```python
from build123d import *

# Parameters (mm, degrees)
EXTRUDE_1_DEPTH      = 50
SKETCH_2_W           = 50
SKETCH_2_H           = 10
EXTRUDE_2_DEPTH      = 10
SKETCH_3_W           = 10
SKETCH_3_H           = 20
EXTRUDE_3_DEPTH      = 20
SKETCH_4_W           = 20
SKETCH_4_H           = 10
EXTRUDE_4_DEPTH      = 30
CUT_EXTRUDE_1_DEPTH  = 50
CHAMFER_1_SIZE       = 2
SKETCH_9_R           = 1.5
CUT_EXTRUDE_2_DEPTH  = 66.493778942
CUT_EXTRUDE_4_DEPTH  = 6
SKETCH_13_W          = 4
SKETCH_13_H          = 6
EXTRUDE_12_DEPTH     = 18
SKETCH_14_W          = 20
SKETCH_14_H          = 20
EXTRUDE_13_DEPTH     = 6
CUT_EXTRUDE_START    = -20
SKETCH_15_W          = 50
SKETCH_15_H          = 6
CUT_EXTRUDE_5_DEPTH  = 20
SKETCH_16_W          = 4
SKETCH_16_H          = 4
CUT_EXTRUDE_7_DEPTH  = 18
EXTRUDE_14_REACH     = 68.163
SKETCH_17_W          = 5
SKETCH_17_H          = 30
SKETCH_18_W          = 50
SKETCH_18_H          = 4
EXTRUDE_15_DEPTH     = 18
CUT_EXTRUDE_8_REACH  = 67.494
SKETCH_19_W          = 60
SKETCH_19_H          = 10
SKETCH_20_R          = 1.5
CUT_EXTRUDE_9_DEPTH  = 4
CHAMFER_2_SIZE       = 2
SKETCH_21_W          = 15
SKETCH_21_H          = 50
CUT_EXTRUDE_10_DEPTH = 10
SKETCH_22_W          = 5
SKETCH_22_H          = 50
EXTRUDE_16_DEPTH     = 19
SKETCH_23_W          = 7
SKETCH_23_H          = 50
CUT_EXTRUDE_11_DEPTH = 4.2
EXTRUDE_17_DEPTH     = 3
SKETCH_25_R          = 1.5
CUT_EXTRUDE_12_DEPTH = 8
SKETCH_26_R          = 2.9
CUT_EXTRUDE_13_DEPTH = 6
CUT_EXTRUDE_14_REACH = 67.988
SKETCH_27_W          = 4
SKETCH_27_H          = 10
SKETCH_29_W          = 8
SKETCH_29_H          = 10
EXTRUDE_18_DEPTH     = 6
SKETCH_30_W          = 50
SKETCH_30_H          = 5
CUT_EXTRUDE_15_DEPTH = 4
EXTRUDE_19_REACH     = 75.219
SKETCH_31_W          = 9.8
SKETCH_31_H          = 10


with BuildPart() as part:
    # 草图1 → 凸台-拉伸1 (new body)
    with BuildSketch(Plane(origin=(0, 0, 0), x_dir=(0, 0, -1), z_dir=(1, 0, 0))):
        Polygon((0, 0), (-10, 0), (-17.716362436, 40), (-12, 41.102738109), (-6, 10), (0, 10), align=None)
    extrude(amount=EXTRUDE_1_DEPTH)

    # 草图2 → 凸台-拉伸2 (add)
    with BuildSketch(Plane.XZ):
        with Locations((25, 5)):
            Rectangle(SKETCH_2_W, SKETCH_2_H)
    extrude(amount=EXTRUDE_2_DEPTH)

    # 草图3 → 凸台-拉伸3 (add)
    with BuildSketch(Plane.ZY):
        with Locations((5, 0)):
            Rectangle(SKETCH_3_W, SKETCH_3_H)
    extrude(amount=EXTRUDE_3_DEPTH)

    # 草图4 → 凸台-拉伸4 (add)
    with BuildSketch(Plane(origin=(0, 10, 0), x_dir=(1, 0, 0), z_dir=(0, 1, 0))):
        with Locations((-10, -5)):
            Rectangle(SKETCH_4_W, SKETCH_4_H)
    extrude(amount=EXTRUDE_4_DEPTH)

    # 草图5 → 切除-拉伸1 (cut)
    with BuildSketch(Plane(origin=(50, 0, 0), x_dir=(0, 0, -1), z_dir=(1, 0, 0))):
        Polygon((-10, 10), (-11.929090609, 10), (-10, 0), align=None)
    extrude(amount=-CUT_EXTRUDE_1_DEPTH, mode=Mode.SUBTRACT)

    # 倒角1
    # the kernel refuses this chamfer: 2 mm, written as the material it adds along each edge
    with BuildSketch(Plane(origin=(50, 10, 10), x_dir=(0, 0.027495876610586487, 0.9996219169112968), z_dir=(-1, 0, 0))) as chamfer_1_piece_1_section:
        Polygon((CHAMFER_1_SIZE * 0.999621916911, -CHAMFER_1_SIZE * 0.0274958766106), (-CHAMFER_1_SIZE * 0.0274958766106, -CHAMFER_1_SIZE * 0.999621916911), (0, 0), align=None)
    chamfer_1_piece_1 = extrude(amount=50, mode=Mode.PRIVATE)
    chamfer_1_piece_1 = split(chamfer_1_piece_1, bisect_by=Plane(origin=(25, 9.122791872, 11.759869213), z_dir=(0, 0.18941678522713282, -0.9818967774029093)), keep=Keep.TOP, mode=Mode.PRIVATE)
    add(chamfer_1_piece_1)

    # 草图9 → 切除-拉伸2 (cut, through all)
    with BuildSketch(Plane.XY.offset(10)):
        with Locations((-10, 30)):
            Circle(SKETCH_9_R)
        with Locations((30, 0)):
            Circle(SKETCH_9_R)
    extrude(amount=-CUT_EXTRUDE_2_DEPTH, mode=Mode.SUBTRACT)

    # 草图12 → 切除-拉伸4 (cut)
    with BuildSketch(Plane.XY.offset(10)):
        Polygon((0, 30.73515874), (0, 40), (-20, 40), (-20, -10), (50, -10), (50, 8), (0, 8), align=None)
    extrude(amount=-CUT_EXTRUDE_4_DEPTH, mode=Mode.SUBTRACT)

    # 草图13 → 凸台-拉伸12 (add)
    with BuildSketch(Plane.XZ.offset(-8)):
        with Locations((2, 7)):
            Rectangle(SKETCH_13_W, SKETCH_13_H)
        with Locations((48, 7)):
            Rectangle(SKETCH_13_W, SKETCH_13_H)
    extrude(amount=EXTRUDE_12_DEPTH)

    # 草图14 → 凸台-拉伸13 (add)
    with BuildSketch(Plane.XY.offset(4)):
        with Locations((-10, 0)):
            Rectangle(SKETCH_14_W, SKETCH_14_H)
    extrude(amount=EXTRUDE_13_DEPTH)

    # 草图15 → 切除-拉伸5 (cut)
    with BuildSketch(Plane(origin=(0, 10, 0), x_dir=(1, 0, 0), z_dir=(0, 1, 0)).offset(CUT_EXTRUDE_START)):
        with Locations((25, -3)):
            Rectangle(SKETCH_15_W, SKETCH_15_H)
    extrude(amount=CUT_EXTRUDE_5_DEPTH, mode=Mode.SUBTRACT)

    # 草图16 → 切除-拉伸7 (cut)
    with BuildSketch(Plane.XZ.offset(10)):
        with Locations((2, 8)):
            Rectangle(SKETCH_16_W, SKETCH_16_H)
        with Locations((48, 8)):
            Rectangle(SKETCH_16_W, SKETCH_16_H)
    extrude(amount=-CUT_EXTRUDE_7_DEPTH, mode=Mode.SUBTRACT)

    # 凸台-拉伸14: up to this plane
    extrude_14_end = Plane(origin=(50, 0, 10), z_dir=(0, 0.1894167852271328, -0.9818967774029093))
    # 草图17 → 凸台-拉伸14 (add, up to the surface)
    with BuildSketch(Plane.XY.offset(4), mode=Mode.PRIVATE) as extrude_14_sk1:
        with Locations((-2.5, 25)):
            Rectangle(SKETCH_17_W, SKETCH_17_H)
    extrude_14_tool1 = split(extrude(extrude_14_sk1.sketch, amount=EXTRUDE_14_REACH, mode=Mode.PRIVATE), bisect_by=extrude_14_end, keep=Keep.BOTH, mode=Mode.PRIVATE)
    add(extrude_14_tool1.solids().sort_by_distance((-2.5, 25, 4))[0])

    # 草图18 → 凸台-拉伸15 (add)
    with BuildSketch(Plane.XZ.offset(-8)):
        with Locations((25, 8)):
            Rectangle(SKETCH_18_W, SKETCH_18_H)
    extrude(amount=EXTRUDE_15_DEPTH)

    # 切除-拉伸8: up to this face of the body (flat: up to its plane)
    cut_extrude_8_end = Plane(part.part.faces().sort_by_distance((-12.539896603, 24.920206795, 4))[0])
    # 草图19 → 切除-拉伸8 (cut, up to the picked face)
    with BuildSketch(Plane.XY.offset(10), mode=Mode.PRIVATE) as cut_extrude_8_sk1:
        with Locations((10, 0)):
            Rectangle(SKETCH_19_W, SKETCH_19_H)
    cut_extrude_8_tool1 = split(extrude(cut_extrude_8_sk1.sketch, amount=-CUT_EXTRUDE_8_REACH, mode=Mode.PRIVATE), bisect_by=cut_extrude_8_end, keep=Keep.BOTH, mode=Mode.PRIVATE)
    add(cut_extrude_8_tool1.solids().sort_by(Axis((10, 0, 10), (0, 0, -1)))[0], mode=Mode.SUBTRACT)

    # 草图20 → 切除-拉伸9 (cut)
    with BuildSketch(Plane.XY.offset(4)):
        with Locations((-10, 0)):
            Circle(SKETCH_20_R)
    extrude(amount=-CUT_EXTRUDE_9_DEPTH, mode=Mode.SUBTRACT)

    # 倒角2
    # the kernel refuses this chamfer: 2 mm, written as the material it adds along each edge
    with BuildSketch(Plane(origin=(5.143365976, 10, 10), x_dir=(0, -0.9996219169112968, -0.027495876610586487), z_dir=(-1, 0, 0))) as chamfer_2_piece_1_section:
        Polygon((CHAMFER_2_SIZE * 0.999621916911, CHAMFER_2_SIZE * 0.0274958766106), (-CHAMFER_2_SIZE * 0.0274958766106, CHAMFER_2_SIZE * 0.999621916911), (0, 0), align=None)
    chamfer_2_piece_1 = extrude(amount=10.143365976, mode=Mode.PRIVATE)
    chamfer_2_piece_1 = split(chamfer_2_piece_1, bisect_by=Plane(origin=(-2.5, 9.121127045, 11.759548053), z_dir=(0, 0.18941678522698793, -0.9818967774029372)), keep=Keep.TOP, mode=Mode.PRIVATE)
    add(chamfer_2_piece_1)

    # 草图21 → 切除-拉伸10 (cut)
    with BuildSketch(Plane.XY.offset(10)):
        with Locations((-12.5, 15)):
            Rectangle(SKETCH_21_W, SKETCH_21_H)
    extrude(amount=-CUT_EXTRUDE_10_DEPTH, mode=Mode.SUBTRACT)

    # 草图22 → 凸台-拉伸16 (add)
    with BuildSketch(Plane(origin=(0, 0, 0), x_dir=(-1, 0, 0), z_dir=(0, 0, -1))):
        with Locations((2.5, 15)):
            Rectangle(SKETCH_22_W, SKETCH_22_H)
    extrude(amount=EXTRUDE_16_DEPTH)

    # 草图23 → 切除-拉伸11 (cut)
    with BuildSketch(Plane(origin=(0, 0, 0), x_dir=(0, 0, -1), z_dir=(1, 0, 0))):
        with Locations((15.5, 15)):
            Rectangle(SKETCH_23_W, SKETCH_23_H)
    extrude(amount=-CUT_EXTRUDE_11_DEPTH, mode=Mode.SUBTRACT)

    # 草图24 → 凸台-拉伸17 (add)
    with BuildSketch(Plane.ZY.offset(5)):
        Polygon((17.716362436, 40), (-19, 40), (-19, -10), (10, -10), (10, -5), (4, -5), (4, 5), (10, 5), (10, 8), (11.912142006, 9.912142006), align=None)
    extrude(amount=EXTRUDE_17_DEPTH)

    # 草图25 → 切除-拉伸12 (cut)
    with BuildSketch(Plane.ZY.offset(8)):
        with Locations(Location((-9, 30, 0), (0, 0, 270))):
            Circle(SKETCH_25_R)
        with Locations(Location((-9, 0, 0), (0, 0, 270))):
            Circle(SKETCH_25_R)
    extrude(amount=-CUT_EXTRUDE_12_DEPTH, mode=Mode.SUBTRACT)

    # 草图26 → 切除-拉伸13 (cut)
    with BuildSketch(Plane.ZY.offset(8)):
        with Locations(Location((-9, 30, 0), (0, 0, 270))):
            Circle(SKETCH_26_R)
        with Locations(Location((-9, 0, 0), (0, 0, 270))):
            Circle(SKETCH_26_R)
    extrude(amount=-CUT_EXTRUDE_13_DEPTH, mode=Mode.SUBTRACT)

    # 草图27 → 切除-拉伸14 (cut, up to next)
    with BuildSketch(Plane.ZY.offset(-40), mode=Mode.PRIVATE) as cut_extrude_14_sk1:
        with Locations((8, 0)):
            Rectangle(SKETCH_27_W, SKETCH_27_H)
    cut_extrude_14_tool1 = extrude(cut_extrude_14_sk1.sketch, amount=-CUT_EXTRUDE_14_REACH, mode=Mode.PRIVATE) & part.part
    add(cut_extrude_14_tool1.solids().sort_by_distance((40, 0, 8))[0], mode=Mode.SUBTRACT)

    # 草图29 → 凸台-拉伸18 (add)
    with BuildSketch(Plane.XY.offset(4)):
        with Locations((-4, 0)):
            Rectangle(SKETCH_29_W, SKETCH_29_H)
    extrude(amount=EXTRUDE_18_DEPTH)

    # 草图30 → 切除-拉伸15 (cut)
    with BuildSketch(Plane.XY.offset(10)):
        with Locations((25, -7.5)):
            Rectangle(SKETCH_30_W, SKETCH_30_H)
    extrude(amount=-CUT_EXTRUDE_15_DEPTH, mode=Mode.SUBTRACT)

    # 凸台-拉伸19: up to this face of the body (flat: up to its plane)
    extrude_19_end = Plane(part.part.faces().sort_by_distance((25, 5, 8))[0])
    # 草图31 → 凸台-拉伸19 (add, up to the picked face)
    with BuildSketch(Plane(origin=(0, 40, 0), x_dir=(1, 0, 0), z_dir=(0, 1, 0)), mode=Mode.PRIVATE) as extrude_19_sk1:
        with Locations((4.9, -7)):
            Rectangle(SKETCH_31_W, SKETCH_31_H)
    extrude_19_tool1 = split(extrude(extrude_19_sk1.sketch, amount=-EXTRUDE_19_REACH, mode=Mode.PRIVATE), bisect_by=extrude_19_end, keep=Keep.BOTH, mode=Mode.PRIVATE)
    add(extrude_19_tool1.solids().sort_by(Axis((4.9, 40, 7), (0, -1, 0)))[0])


solid = part.part
```
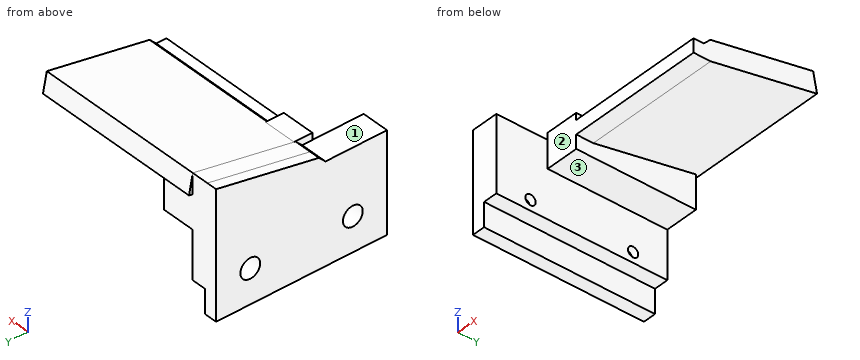
Verification items for the finished model (mm, model axes). Face numbers are marked on the shaded views. A direction names the side the tool comes from. Give positions to 0.01 mm unless a question says otherwise; leave off trailing zeros. Order: outer loops, then holes, each group sorted by start corner. A loop starts at its lowest first (then second) coordinate and runs counter-clockwise, first axis right, second up. Notation, with made-up numbers: (14, 51) -> (62, 51) arc R23 cw to (62, 72) -> close; hole circle Ø8 at (72.5, 56.25). An arc over 180 degrees is marked (long way). Use a Markdown table: item, result.
1) Depth check by flat-ended pin: pin 1 Ø4 at (y, z) = (-3, 13.5) entering from -X; pin 2 Ø11 at (x, z) = (19, 5) entering from -Y; pin 3 Ø6 at (x, y) = (6, 8) entering from +Z; pin 4 Ø0.9 at (y, z) = (40.5, 16) entering from -X. Enter the tip coordinate at first touch or a pass-through.
Results:
| item | result |
|---|---|
| pin 1 | through |
| pin 2 | y = 5 |
| pin 3 | z = 12.12 |
| pin 4 | x = 0 |
2) Section check B-B, the plane z = -9. Record the boundary of the cut face in (x, y), then the cut area to 3 significant figures.
Results:
| item | result |
|---|---|
| outline | (-8, -10) -> (0, -10) -> (0, -1.5) -> (-2, -1.5) -> (-2, -2.9) -> (-8, -2.9) -> close; (-8, 2.9) -> (-2, 2.9) -> (-2, 1.5) -> (0, 1.5) -> (0, 28.5) -> (-2, 28.5) -> (-2, 27.1) -> (-8, 27.1) -> close; (-8, 32.9) -> (-2, 32.9) -> (-2, 31.5) -> (0, 31.5) -> (0, 40) -> (-8, 40) -> close |
| area | 318 mm² |
3) Section check D-D, the plane z = 3.5. Record the boundary of the cut face in (x, y).
Results:
| item | result |
|---|---|
| outline | (-8, -10) -> (0, -10) -> (0, 5) -> (9.8, 5) -> (9.8, 40) -> (-8, 40) -> close |
4) Section check A-A, the plane y = 0. Record the boundary of the cut face in (x, z), then the cut area to 3 significant figures.
Results:
| item | result |
|---|---|
| outline | (-8, -19) -> (-4.2, -19) -> (-4.2, -12) -> (0, -12) -> (0, -10.5) -> (-2, -10.5) -> (-2, -11.9) -> (-8, -11.9) -> close; (-8, -6.1) -> (-2, -6.1) -> (-2, -7.5) -> (0, -7.5) -> (0, 10) -> (-8, 10) -> close |
| area | 162 mm² |
5) Section check C-C, the plane x = 36. Record the boundary of the cut face in (y, z).
Results:
| item | result |
|---|---|
| outline | (5, 6) -> (10, 6) -> (41.1, 12) -> (40, 17.72) -> (9.91, 11.91) -> (8, 10) -> (5, 10) -> close |
6) Material ranges on probe 1 along Z at (x, y) = (-1, 0); probe 2 along Z at (x, y) = (-5.3, 30); probe 3 along Y at (x, z) = (-2.5, -10), recorded low to high.
Results:
| item | result |
|---|---|
| probe 1 | -12 to -10.5, -7.5 to 10 |
| probe 2 | -19 to -11.9, -6.1 to 15.79 |
| probe 3 | -10 to -2.72, 2.72 to 27.28, 32.72 to 40 |
7) Tool access check on the marked faces 1, 2 and 3. Record the directions out of +Z, -Z, +X, -X, +Y, -Y that give a thin tool (end or side, any length) a straight path to the whole face; none if there is none.
Results:
| item | result |
|---|---|
| face 1 | +Z, -X, -Y |
| face 2 | +Z, -Z, +X, -Y |
| face 3 | -Z, +X, +Y, -Y |
